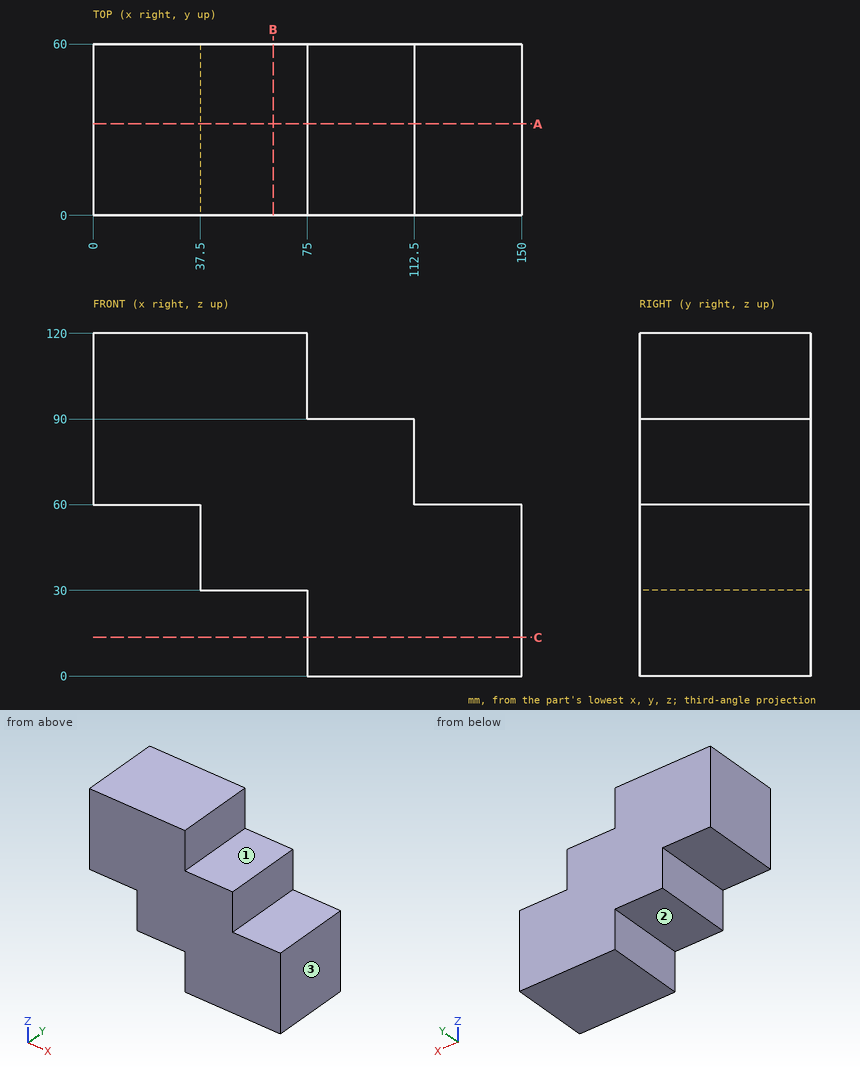
Print and shaded views of the part. All mm, measured from the part's lowest x, y and z. A direction names the side the tool comes from. Coordinates: 2 decimals unless noted, no trailing zeros. Loops run counter-clockwise (first coordinate to the right, second up) from the corner with the lowest first, then second, coordinate; pieces in that order, holes last. Notation, with made-up numbers: (70.25, -35.5) -> (128.25, -35.5) arc R30 ccw to (128.25, -0.5) -> close; hole circle Ø4 at (-6.75, 73.5). An arc over 180 degrees is marked (long way). Use a Markdown table: item, result. Add a question column.
Item 1: Probe probe 1 along Z at (x, y) = (49.5, 20.5); probe 2 along Z at (x, y) = (91.5, 56); probe 3 along X at (y, z) = (24, 89). List the from-to ranges inside material, lowest first.
Item 2: Which spindle directions (+Z, -Z, +X, -X, +Y, -Y) get a long thin tool onto all of the face, cutting with end or side? Do the marked faces 1, 2 and 3. Say none if no direction does.
Item 3: Flat gauge pins, fed straight in: P1, Ø11, axis at x = 128, y = 35, coming from the +Z side; P2, Ø3, axis at x = 96, y = 38, coming from the +Z side; P3, Ø9, axis at y = 21.5, z = 71.5, coming from the +X side; P4, Ø1, axis at y = 39, z = 93.5, coming from the -X side. Where does each tip first touch, or does it go through?
Item 4: Band-saw the part on C-C on z = 13.5. Write the cut outline in (x, y).
Item 5: Band-saw the part on A-A on y = 32. Write the cut outline in (x, z).
Item 6: Band-saw the part on B-B on x = 63. Write the cut outline in (y, z), plus the area to 3 significant figures.
Geometry says:
| question | item | result |
|---|---|---|
| 1 | probe 1 | 30 to 120 |
| 1 | probe 2 | 0 to 90 |
| 1 | probe 3 | 0 to 112.5 |
| 2 | face 1 | +Z, +X, +Y, -Y |
| 2 | face 2 | -Z, -X, +Y, -Y |
| 2 | face 3 | +Z, -Z, +X, +Y, -Y |
| 3 | P1 | z = 60 |
| 3 | P2 | z = 90 |
| 3 | P3 | x = 112.5 |
| 3 | P4 | x = 0 |
| 4 | outline | (75, 0) -> (150, 0) -> (150, 60) -> (75, 60) -> close |
| 5 | outline | (0, 60) -> (37.5, 60) -> (37.5, 30) -> (75, 30) -> (75, 0) -> (150, 0) -> (150, 60) -> (112.5, 60) -> (112.5, 90) -> (75, 90) -> (75, 120) -> (0, 120) -> close |
| 6 | outline | (0, 30) -> (60, 30) -> (60, 120) -> (0, 120) -> close |
| 6 | area | 5,400 mm² |
